Build history of the part. All positions in model axes, mm. A direction names the side the tool comes from. Give positions to 0.01 mm unless a question says otherwise; leave off trailing zeros. Order: outer loops, then holes, each group sorted by start corner. A loop starts at its lowest first (then second) coordinate and runs counter-clockwise, first axis right, second up. Notation, with made-up numbers: (20, 6) - (54, 6) arc R21 ccw to (54, 27) - close; hole circle Ø9 at (13.5, -17.75). An arc over 180 degrees is marked (long way). Answer in a Markdown table with one row per item.
```python
from build123d import *

# Parameters (mm, degrees)
BOSS_EXTRUDE2_DEPTH        = 12.7
F_1_1_DIAMETER_HOLE1_D     = 25.4
SKETCH6_W                  = 63.5
SKETCH6_H                  = 25.4
CUT_EXTRUDE1_DEPTH         = 12.7
SKETCH7_W                  = 31.75
SKETCH7_H                  = 12.7
CUT_EXTRUDE2_DEPTH         = 12.7
SKETCH8_W                  = 31.75
SKETCH8_H                  = 12.7
BOSS_EXTRUDE3_DEPTH        = 28.575
F_1_2_0_5_DIAMETER_HOLE1_D = 12.7
CUT_EXTRUDE4_DEPTH         = 12.7


with BuildPart() as part:
    # Sketch3 → Boss-Extrude2 (new body)
    with BuildSketch(Plane(origin=(0, 0, 0), x_dir=(1, 0, 0), z_dir=(0, 1, 0))):
        with BuildLine():
            Line((0, 0), (-63.5, 0))
            ThreePointArc((-63.5, 0), (-88.9, 25.4), (-63.5, 50.8))
            Line((-63.5, 50.8), (0, 50.8))
            ThreePointArc((0, 50.8), (25.4, 25.4), (0, 0))
        make_face()
    extrude(amount=BOSS_EXTRUDE2_DEPTH)

    # 1 (1) Diameter Hole1 (through all)
    with Locations(Plane(origin=(0, 12.7, 0), x_dir=(1, 0, 0), z_dir=(0, 1, 0))):
        with Locations((-63.5, 25.4), (0, 25.4)):
            Hole(F_1_1_DIAMETER_HOLE1_D / 2)

    # Sketch6 → Cut-Extrude1 (cut)
    with BuildSketch(Plane(origin=(0, 12.7, 0), x_dir=(1, 0, 0), z_dir=(0, 1, 0))):
        with Locations((-31.75, 25.4)):
            Rectangle(SKETCH6_W, SKETCH6_H)
    extrude(amount=-CUT_EXTRUDE1_DEPTH, mode=Mode.SUBTRACT)

    # Sketch7 → Cut-Extrude2 (cut)
    with BuildSketch(Plane.XY):
        with Locations((-31.75, 6.35)):
            Rectangle(SKETCH7_W, SKETCH7_H)
    extrude(amount=-CUT_EXTRUDE2_DEPTH, mode=Mode.SUBTRACT)

    # Sketch8 → Boss-Extrude3 (add)
    with BuildSketch(Plane(origin=(0, 12.7, 0), x_dir=(1, 0, 0), z_dir=(0, 1, 0))):
        with Locations((-31.75, 44.45)):
            Rectangle(SKETCH8_W, SKETCH8_H)
    extrude(amount=BOSS_EXTRUDE3_DEPTH)

    # 1/2 (0.5) Diameter Hole1 (through all)
    with Locations(Plane.XY.offset(-38.1)):
        with Locations((-31.75, 25.4)):
            Hole(F_1_2_0_5_DIAMETER_HOLE1_D / 2)

    # Sketch12 → Cut-Extrude4 (cut)
    with BuildSketch(Plane.XY.offset(-38.1)):
        with BuildLine():
            Line((-31.75, 41.275), (-47.625, 41.275))
            Line((-47.625, 41.275), (-47.625, 25.4))
            ThreePointArc((-47.625, 25.4), (-42.975320151, 36.625320151), (-31.75, 41.275))
        make_face()
        with BuildLine():
            Line((-15.875, 41.275), (-31.75, 41.275))
            ThreePointArc((-31.75, 41.275), (-20.524679849, 36.625320151), (-15.875, 25.4))
            Line((-15.875, 25.4), (-15.875, 41.275))
        make_face()
    extrude(amount=-CUT_EXTRUDE4_DEPTH, mode=Mode.SUBTRACT)


solid = part.part
```
1. Two-plate mould, pull along Z, no slides. Class faces 1 (the face through (-47.625, 6, -6)), 2 (the face through (-8, 6, 0)), 3 (the face through (-76.197, 6.261, -25.121)): +Z half, -Z half, draft (parallel to the pull), parting line (faces both ways), or undercut.
Check result:
| item | result |
|---|---|
| face 1 | draft |
| face 2 | +Z half |
| face 3 | undercut |
2. Cut at B-B on x = -4. Write the cut outline in (y, z).
Check result:
| item | result |
|---|---|
| outline | (0, -50.8) - (12.7, -50.8) - (12.7, -38.1) - (0, -38.1) - close; (0, -12.7) - (12.7, -12.7) - (12.7, 0) - (0, 0) - close |
3. Which spindle directions (+Z, -Z, +X, -X, +Y, -Y) get a long thin tool onto all of the face, cutting with end or side? Do faces 4 (the face through (-8, 6, -12.7)), 5 (the face through (-15.875, 6, -6)), 6 (the face through (-88.894, 6.261, -24.841)), 7 (the face through (-77, 12.7, -26)), 8 (the face through (-15.875, 19, -44)). Say none if no direction does.
Check result:
| item | result |
|---|---|
| face 4 | +Y, -Y |
| face 5 | +Z, +Y, -Y |
| face 6 | -X, +Y, -Y |
| face 7 | +Z, -Z, -X, +Y |
| face 8 | +Z, -Z, +X, +Y |
4. Cut at D-D on x = -43.5. Write the cut outline in (y, z), and give its area (3 significant figures).
Check result:
| item | result |
|---|---|
| outline | (0, -50.8) - (36.07, -50.8) - (36.07, -38.1) - (0, -38.1) - close |
| area | 458 mm² |
5. Drop flat-ended pins along their axis: P1, Ø4, axis at y = 4, z = -4, coming from the +X side; P2, Ø10, axis at y = 19.5, z = -42.5, coming from the +X side (3 decimals); P3, Ø4, axis at x = 6, z = -41, coming from the +Y side; P4, Ø2, axis at x = 9, z = -21.5, coming from the +Y side. Give the stop position or say it passes through.
Check result:
| item | result |
|---|---|
| P1 | stops at x = 16.4 |
| P2 | stops at x = -15.875 |
| P3 | stops at y = 12.7 |
| P4 | passes through |
6. Cut at C-C on y = 4. Write the cut outline in (x, z) (3 decimals).
Check result:
| item | result |
|---|---|
| outline | (-63.5, -50.8) - (0, -50.8) arc R25.4 ccw to (0, 0) - (-15.875, 0) - (-15.875, -12.7) - (0, -12.7) arc R12.7 cw to (0, -38.1) - (-63.5, -38.1) arc R12.7 cw to (-63.5, -12.7) - (-47.625, -12.7) - (-47.625, 0) - (-63.5, 0) arc R25.4 ccw to start |
7. Cut at A-A on z = -23.5. Write the cut outline in (x, y), and give its area (3 significant figures).
Check result:
| item | result |
|---|---|
| outline | (-88.83, 0) - (-76.06, 0) - (-76.06, 12.7) - (-88.83, 12.7) - close; (12.56, 0) - (25.33, 0) - (25.33, 12.7) - (12.56, 12.7) - close |
| area | 324 mm² |
8. Probe line 1 (Y direction, x = -31.75, z = -47.5) (3 decimals); line 2 (Y direction, x = -81.5, z = -15); line 3 (Z direction, x = -25, y = 38). List the from-to ranges inside material, lowest first.
Check result:
| item | result |
|---|---|
| line 1 | y = 0 to 19.05, 31.75 to 41.275 |
| line 2 | y = 0 to 12.7 |
| line 3 | z = -50.8 to -38.1 |
